from build123d import *

# Parameters (mm, degrees)
SKETCH1_R                 = 10.5
SKETCH1_R_2               = 1.5
SKETCH1_W                 = 8
SKETCH1_H                 = 40
SKETCH1_R_3               = 17.5
BOSS_EXTRUDE1_DEPTH       = 3
CUT_EXTRUDE1_REACH        = 140.687
SKETCH2_R                 = 2
CUT_EXTRUDE2_REACH        = 140.687
SKETCH3_R                 = 2
BOSS_EXTRUDE2_START       = -3
SKETCH4_R                 = 65
SKETCH4_R_2               = 60
BOSS_EXTRUDE2_DEPTH       = 3
CUT_EXTRUDE3_START        = -10
CUT_EXTRUDE3_DEPTH        = 10
CUT_EXTRUDE4_START        = -10
CUT_EXTRUDE4_DEPTH        = 10
CUT_EXTRUDE5_REACH        = 142.922
SKETCH7_R                 = 1.5
CUT_EXTRUDE6_REACH        = 142.922
SKETCH8_R                 = 1.5
CUT_EXTRUDE7_REACH        = 142.922
SKETCH9_R                 = 1.5
F_3_0MM_DOWEL_HOLE1_D     = 3
F_3_0MM_DOWEL_HOLE1_DEPTH = 11.3
F_3_0MM_DOWEL_HOLE1_TIP   = 0.901290929
CUT_EXTRUDE8_REACH        = 142.922
SKETCH13_R                = 1


with BuildPart() as part:
    # Sketch1 → Boss-Extrude1 (new body)
    # profile 1 of 2: a face of its own
    with BuildSketch(Plane.XY):
        with BuildLine():
            ThreePointArc((-60, 0), (-52.867640737, 28.372743309), (-33.166247904, 50))
            Line((-33.166247904, 50), (-60, 50))
            Line((-60, 50), (-60, 0))
        make_face()
    # profile 2 of 2: a face of its own
    with BuildSketch(Plane.XY):
        with BuildLine():
            ThreePointArc((0, 60), (-17.320508076, 57.445626465), (-33.166247904, 50))
            ThreePointArc((-33.166247904, 50), (-52.867640737, 28.372743309), (-60, 0))
            ThreePointArc((-60, 0), (-15.529142706, -57.955549577), (51.961524227, -30))
            Line((51.961524227, -30), (56.568542495, -30))
            Line((56.568542495, -30), (90, -30))
            Line((90, -30), (90, -10.355339059))
            Line((90, -10.355339059), (117.67766953, 17.32233047))
            ThreePointArc((117.67766953, 17.32233047), (123.096988313, 44.567085809), (100, 60))
            Line((100, 60), (0, 60))
        make_face()
        Circle(SKETCH1_R, mode=Mode.SUBTRACT)
        with Locations((69, -26)):
            Circle(SKETCH1_R_2, mode=Mode.SUBTRACT)
        with Locations((76, 0)):
            Rectangle(SKETCH1_W, SKETCH1_H, mode=Mode.SUBTRACT)
        with Locations((83, -26)):
            Circle(SKETCH1_R_2, mode=Mode.SUBTRACT)
        with Locations((100, 35)):
            Circle(SKETCH1_R_3, mode=Mode.SUBTRACT)
    extrude(amount=BOSS_EXTRUDE1_DEPTH)

    # Sketch2 → Cut-Extrude1 (cut, up to next)
    with BuildSketch(Plane.XY.offset(3), mode=Mode.PRIVATE) as cut_extrude1_sk1:
        with Locations((60, 45)):
            Circle(SKETCH2_R)
    cut_extrude1_tool1 = extrude(cut_extrude1_sk1.sketch, amount=-CUT_EXTRUDE1_REACH, mode=Mode.PRIVATE) & part.part
    add(cut_extrude1_tool1.solids().sort_by_distance((60, 45, 3))[0], mode=Mode.SUBTRACT)

    # Sketch3 → Cut-Extrude2 (cut, up to next)
    with BuildSketch(Plane.XY.offset(3), mode=Mode.PRIVATE) as cut_extrude2_sk1:
        with Locations((100, 10)):
            Circle(SKETCH3_R)
    cut_extrude2_tool1 = extrude(cut_extrude2_sk1.sketch, amount=-CUT_EXTRUDE2_REACH, mode=Mode.PRIVATE) & part.part
    # Sketch3 → Cut-Extrude2 (cut, up to next)
    with BuildSketch(Plane.XY.offset(3), mode=Mode.PRIVATE) as cut_extrude2_sk2:
        with Locations((75, 35)):
            Circle(SKETCH3_R)
    cut_extrude2_tool2 = extrude(cut_extrude2_sk2.sketch, amount=-CUT_EXTRUDE2_REACH, mode=Mode.PRIVATE) & part.part
    # Sketch3 → Cut-Extrude2 (cut, up to next)
    with BuildSketch(Plane.XY.offset(3), mode=Mode.PRIVATE) as cut_extrude2_sk3:
        with Locations((115.0260191, 50.0260191)):
            Circle(SKETCH3_R)
    cut_extrude2_tool3 = extrude(cut_extrude2_sk3.sketch, amount=-CUT_EXTRUDE2_REACH, mode=Mode.PRIVATE) & part.part
    add(cut_extrude2_tool1.solids().sort_by_distance((100, 10, 3))[0], mode=Mode.SUBTRACT)
    add(cut_extrude2_tool2.solids().sort_by_distance((75, 35, 3))[0], mode=Mode.SUBTRACT)
    add(cut_extrude2_tool3.solids().sort_by_distance((115.026019, 50.026019, 3))[0], mode=Mode.SUBTRACT)

    # Sketch4 → Boss-Extrude2 (add)
    with BuildSketch(Plane.XY.offset(3).offset(BOSS_EXTRUDE2_START)):
        Circle(SKETCH4_R)
        Circle(SKETCH4_R_2, mode=Mode.SUBTRACT)
    extrude(amount=BOSS_EXTRUDE2_DEPTH)

    # Sketch5 → Cut-Extrude3 (cut)
    with BuildSketch(Plane.XY.offset(3).offset(CUT_EXTRUDE3_START)):
        with BuildLine():
            Line((-60, 50), (-41.533119315, 50))
            ThreePointArc((-41.533119315, 50), (-52.282822987, 38.62002616), (-60, 25))
            Line((-60, 25), (-60, 50))
        make_face()
    extrude(amount=CUT_EXTRUDE3_DEPTH, mode=Mode.SUBTRACT)

    # Sketch6 → Cut-Extrude4 (cut)
    with BuildSketch(Plane.XY.offset(3).offset(CUT_EXTRUDE4_START)):
        with BuildLine():
            Line((25, 60), (-25, 60))
            ThreePointArc((-25, 60), (0, 65), (25, 60))
        make_face()
    extrude(amount=CUT_EXTRUDE4_DEPTH, mode=Mode.SUBTRACT)

    # Sketch7 → Cut-Extrude5 (cut, up to next)
    with BuildSketch(Plane.XY.offset(3), mode=Mode.PRIVATE) as cut_extrude5_sk1:
        with Locations((-14.5, 12)):
            Circle(SKETCH7_R)
    cut_extrude5_tool1 = extrude(cut_extrude5_sk1.sketch, amount=-CUT_EXTRUDE5_REACH, mode=Mode.PRIVATE) & part.part
    # Sketch7 → Cut-Extrude5 (cut, up to next)
    with BuildSketch(Plane.XY.offset(3), mode=Mode.PRIVATE) as cut_extrude5_sk2:
        with Locations((14.5, 12)):
            Circle(SKETCH7_R)
    cut_extrude5_tool2 = extrude(cut_extrude5_sk2.sketch, amount=-CUT_EXTRUDE5_REACH, mode=Mode.PRIVATE) & part.part
    # Sketch7 → Cut-Extrude5 (cut, up to next)
    with BuildSketch(Plane.XY.offset(3), mode=Mode.PRIVATE) as cut_extrude5_sk3:
        with Locations((-14.5, -12)):
            Circle(SKETCH7_R)
    cut_extrude5_tool3 = extrude(cut_extrude5_sk3.sketch, amount=-CUT_EXTRUDE5_REACH, mode=Mode.PRIVATE) & part.part
    # Sketch7 → Cut-Extrude5 (cut, up to next)
    with BuildSketch(Plane.XY.offset(3), mode=Mode.PRIVATE) as cut_extrude5_sk4:
        with Locations((14.5, -12)):
            Circle(SKETCH7_R)
    cut_extrude5_tool4 = extrude(cut_extrude5_sk4.sketch, amount=-CUT_EXTRUDE5_REACH, mode=Mode.PRIVATE) & part.part
    add(cut_extrude5_tool1.solids().sort_by_distance((-14.5, 12, 3))[0], mode=Mode.SUBTRACT)
    add(cut_extrude5_tool2.solids().sort_by_distance((14.5, 12, 3))[0], mode=Mode.SUBTRACT)
    add(cut_extrude5_tool3.solids().sort_by_distance((-14.5, -12, 3))[0], mode=Mode.SUBTRACT)
    add(cut_extrude5_tool4.solids().sort_by_distance((14.5, -12, 3))[0], mode=Mode.SUBTRACT)

    # Sketch8 → Cut-Extrude6 (cut, up to next)
    with BuildSketch(Plane.XY.offset(3), mode=Mode.PRIVATE) as cut_extrude6_sk1:
        with Locations((50, 38)):
            Circle(SKETCH8_R)
    cut_extrude6_tool1 = extrude(cut_extrude6_sk1.sketch, amount=-CUT_EXTRUDE6_REACH, mode=Mode.PRIVATE) & part.part
    # Sketch8 → Cut-Extrude6 (cut, up to next)
    with BuildSketch(Plane.XY.offset(3), mode=Mode.PRIVATE) as cut_extrude6_sk2:
        with Locations((13, 38)):
            Circle(SKETCH8_R)
    cut_extrude6_tool2 = extrude(cut_extrude6_sk2.sketch, amount=-CUT_EXTRUDE6_REACH, mode=Mode.PRIVATE) & part.part
    # Sketch8 → Cut-Extrude6 (cut, up to next)
    with BuildSketch(Plane.XY.offset(3), mode=Mode.PRIVATE) as cut_extrude6_sk3:
        with Locations((50, -31)):
            Circle(SKETCH8_R)
    cut_extrude6_tool3 = extrude(cut_extrude6_sk3.sketch, amount=-CUT_EXTRUDE6_REACH, mode=Mode.PRIVATE) & part.part
    # Sketch8 → Cut-Extrude6 (cut, up to next)
    with BuildSketch(Plane.XY.offset(3), mode=Mode.PRIVATE) as cut_extrude6_sk4:
        with Locations((13, -31)):
            Circle(SKETCH8_R)
    cut_extrude6_tool4 = extrude(cut_extrude6_sk4.sketch, amount=-CUT_EXTRUDE6_REACH, mode=Mode.PRIVATE) & part.part
    # Sketch8 → Cut-Extrude6 (cut, up to next)
    with BuildSketch(Plane.XY.offset(3), mode=Mode.PRIVATE) as cut_extrude6_sk5:
        with Locations((-5, 34)):
            Circle(SKETCH8_R)
    cut_extrude6_tool5 = extrude(cut_extrude6_sk5.sketch, amount=-CUT_EXTRUDE6_REACH, mode=Mode.PRIVATE) & part.part
    # Sketch8 → Cut-Extrude6 (cut, up to next)
    with BuildSketch(Plane.XY.offset(3), mode=Mode.PRIVATE) as cut_extrude6_sk6:
        with Locations((-32.9, 34)):
            Circle(SKETCH8_R)
    cut_extrude6_tool6 = extrude(cut_extrude6_sk6.sketch, amount=-CUT_EXTRUDE6_REACH, mode=Mode.PRIVATE) & part.part
    # Sketch8 → Cut-Extrude6 (cut, up to next)
    with BuildSketch(Plane.XY.offset(3), mode=Mode.PRIVATE) as cut_extrude6_sk7:
        with Locations((0.1, -18.1)):
            Circle(SKETCH8_R)
    cut_extrude6_tool7 = extrude(cut_extrude6_sk7.sketch, amount=-CUT_EXTRUDE6_REACH, mode=Mode.PRIVATE) & part.part
    # Sketch8 → Cut-Extrude6 (cut, up to next)
    with BuildSketch(Plane.XY.offset(3), mode=Mode.PRIVATE) as cut_extrude6_sk8:
        with Locations((-48.1, -16.8)):
            Circle(SKETCH8_R)
    cut_extrude6_tool8 = extrude(cut_extrude6_sk8.sketch, amount=-CUT_EXTRUDE6_REACH, mode=Mode.PRIVATE) & part.part
    add(cut_extrude6_tool1.solids().sort_by_distance((50, 38, 3))[0], mode=Mode.SUBTRACT)
    add(cut_extrude6_tool2.solids().sort_by_distance((13, 38, 3))[0], mode=Mode.SUBTRACT)
    add(cut_extrude6_tool3.solids().sort_by_distance((50, -31, 3))[0], mode=Mode.SUBTRACT)
    add(cut_extrude6_tool4.solids().sort_by_distance((13, -31, 3))[0], mode=Mode.SUBTRACT)
    add(cut_extrude6_tool5.solids().sort_by_distance((-5, 34, 3))[0], mode=Mode.SUBTRACT)
    add(cut_extrude6_tool6.solids().sort_by_distance((-32.9, 34, 3))[0], mode=Mode.SUBTRACT)
    add(cut_extrude6_tool7.solids().sort_by_distance((0.1, -18.1, 3))[0], mode=Mode.SUBTRACT)
    add(cut_extrude6_tool8.solids().sort_by_distance((-48.1, -16.8, 3))[0], mode=Mode.SUBTRACT)

    # Sketch9 → Cut-Extrude7 (cut, up to next)
    with BuildSketch(Plane.XY.offset(3), mode=Mode.PRIVATE) as cut_extrude7_sk1:
        with Locations((-21.3, -26.2)):
            Circle(SKETCH9_R)
    cut_extrude7_tool1 = extrude(cut_extrude7_sk1.sketch, amount=-CUT_EXTRUDE7_REACH, mode=Mode.PRIVATE) & part.part
    # Sketch9 → Cut-Extrude7 (cut, up to next)
    with BuildSketch(Plane.XY.offset(3), mode=Mode.PRIVATE) as cut_extrude7_sk2:
        with Locations((-21.2, 20)):
            Circle(SKETCH9_R)
    cut_extrude7_tool2 = extrude(cut_extrude7_sk2.sketch, amount=-CUT_EXTRUDE7_REACH, mode=Mode.PRIVATE) & part.part
    # Sketch9 → Cut-Extrude7 (cut, up to next)
    with BuildSketch(Plane.XY.offset(3), mode=Mode.PRIVATE) as cut_extrude7_sk3:
        with Locations((-45, 20)):
            Circle(SKETCH9_R)
    cut_extrude7_tool3 = extrude(cut_extrude7_sk3.sketch, amount=-CUT_EXTRUDE7_REACH, mode=Mode.PRIVATE) & part.part
    # Sketch9 → Cut-Extrude7 (cut, up to next)
    with BuildSketch(Plane.XY.offset(3), mode=Mode.PRIVATE) as cut_extrude7_sk4:
        with Locations((-44.9, -26.2)):
            Circle(SKETCH9_R)
    cut_extrude7_tool4 = extrude(cut_extrude7_sk4.sketch, amount=-CUT_EXTRUDE7_REACH, mode=Mode.PRIVATE) & part.part
    add(cut_extrude7_tool1.solids().sort_by_distance((-21.3, -26.2, 3))[0], mode=Mode.SUBTRACT)
    add(cut_extrude7_tool2.solids().sort_by_distance((-21.2, 20, 3))[0], mode=Mode.SUBTRACT)
    add(cut_extrude7_tool3.solids().sort_by_distance((-45, 20, 3))[0], mode=Mode.SUBTRACT)
    add(cut_extrude7_tool4.solids().sort_by_distance((-44.9, -26.2, 3))[0], mode=Mode.SUBTRACT)

    # Ø3.0mm Dowel Hole1
    with Locations(Plane.XY.offset(3)):
        with Locations((44, 0)):
            Hole(F_3_0MM_DOWEL_HOLE1_D / 2, depth=F_3_0MM_DOWEL_HOLE1_DEPTH)
            with Locations((0, 0, -(F_3_0MM_DOWEL_HOLE1_DEPTH + F_3_0MM_DOWEL_HOLE1_TIP / 2))):  # 118° drill point
                Cone(0, F_3_0MM_DOWEL_HOLE1_D / 2, F_3_0MM_DOWEL_HOLE1_TIP, mode=Mode.SUBTRACT)

    # Sketch13 → Cut-Extrude8 (cut, up to next)
    with BuildSketch(Plane.XY.offset(3), mode=Mode.PRIVATE) as cut_extrude8_sk1:
        with Locations((-40.478838325, 29.696152423)):
            Circle(SKETCH13_R)
    cut_extrude8_tool1 = extrude(cut_extrude8_sk1.sketch, amount=-CUT_EXTRUDE8_REACH, mode=Mode.PRIVATE) & part.part
    # Sketch13 → Cut-Extrude8 (cut, up to next)
    with BuildSketch(Plane.XY.offset(3), mode=Mode.PRIVATE) as cut_extrude8_sk2:
        with Locations((-33.978838325, 29.696152423)):
            Circle(SKETCH13_R)
    cut_extrude8_tool2 = extrude(cut_extrude8_sk2.sketch, amount=-CUT_EXTRUDE8_REACH, mode=Mode.PRIVATE) & part.part
    # Sketch13 → Cut-Extrude8 (cut, up to next)
    with BuildSketch(Plane.XY.offset(3), mode=Mode.PRIVATE) as cut_extrude8_sk3:
        with Locations((8, -38.4)):
            Circle(SKETCH13_R)
    cut_extrude8_tool3 = extrude(cut_extrude8_sk3.sketch, amount=-CUT_EXTRUDE8_REACH, mode=Mode.PRIVATE) & part.part
    # Sketch13 → Cut-Extrude8 (cut, up to next)
    with BuildSketch(Plane.XY.offset(3), mode=Mode.PRIVATE) as cut_extrude8_sk4:
        with Locations((8, -44.9)):
            Circle(SKETCH13_R)
    cut_extrude8_tool4 = extrude(cut_extrude8_sk4.sketch, amount=-CUT_EXTRUDE8_REACH, mode=Mode.PRIVATE) & part.part
    add(cut_extrude8_tool1.solids().sort_by_distance((-40.478838, 29.696152, 3))[0], mode=Mode.SUBTRACT)
    add(cut_extrude8_tool2.solids().sort_by_distance((-33.978838, 29.696152, 3))[0], mode=Mode.SUBTRACT)
    add(cut_extrude8_tool3.solids().sort_by_distance((8, -38.4, 3))[0], mode=Mode.SUBTRACT)
    add(cut_extrude8_tool4.solids().sort_by_distance((8, -44.9, 3))[0], mode=Mode.SUBTRACT)


solid = part.part
Design review of the part built by this model. Coordinates are the model's own, in mm. Give positions to 0.01 mm unless a question says otherwise; leave off trailing zeros. Order: outer loops, then holes, each group sorted by start corner. A loop starts at its lowest first (then second) coordinate and runs counter-clockwise, first axis right, second up. Notation, with made-up numbers: (-39, -17) - (-15, -17) arc R22 ccw to (-15, 15) - close; hole circle Ø7 at (47.25, 20). An arc over 180 degrees is marked (long way). Write item = value, one per line. Start each with the question number.
Q1. We need section C-C on z = 0.9. State how many separate pieces and enclosed holes the cut face has, plus the area to 3 significant figures.
Q2. We need section A-A on y = 45. State the section outline as (x, z) points, plus the area to 3 significant figures.
Q3. We need section D-D on x = 37. State the section outline as (y, z) points, plus the area to 3 significant figures.
Q4. To check wall thickness, follow L1, parallel to Y at x = -22.5, z = 2.1; L2, parallel to Y at x = 100, z = 1.65; L3, parallel to X at y = 20.5, z = 1.45. State the ranges of each line that lie inside material, in increasing order. Write a range as from..to.
Q5. Clearance check with flat-ended pins moving along their axes: pin 1 Ø2.5 at (x, y) = (50, 38) entering from -Z; pin 2 Ø1 at (y, z) = (14.5, 2.5) entering from +X; pin 3 Ø1 at (y, z) = (-3.5, 1.5) entering from +X. State where each tip first meets the part, or that it passes through.
Q6. We need section B-B on x = 95.5. State the section outline as (y, z) points, plus the area to 3 significant figures.
Working result:
q1.separate_pieces = 1
q1.enclosed_holes = 30
q1.area = 16,000 mm²
q2.outline = (-46.9, 0) - (58, 0) - (58, 3) - (-46.9, 3) - close; (62, 0) - (85.64, 0) - (85.64, 3) - (62, 3) - close; (114.36, 0) - (122.91, 0) - (122.91, 3) - (114.36, 3) - close
q2.area = 411 mm²
q3.outline = (-53.44, 0) - (60, 0) - (60, 3) - (-53.44, 3) - close
q3.area = 340 mm²
q4.L1 = -60.98..-27.1, -25.3..19.25, 20.75..60
q4.L2 = -0.36..8, 12..17.5, 52.5..60
q4.L3 = -61.68..-46.41, -43.59..-22.61, -19.79..90.2, 109.8..120.37
q5.pin_1 = through
q5.pin_2 = 115.36
q5.pin_3 = 97.36
q6.outline = (-4.86, 0) - (18.09, 0) - (18.09, 3) - (-4.86, 3) - close; (51.91, 0) - (60, 0) - (60, 3) - (51.91, 3) - close
q6.area = 93.1 mm²
